Read the model definition and answer for the solid it produces. Units are mm, in the model's axes. A direction names the side the tool comes from. Round coordinates to 2 decimals unless told otherwise and drop trailing zeros. Order: outer loops, then holes, each group sorted by start corner. A loop starts at its lowest first (then second) coordinate and runs counter-clockwise, first axis right, second up. Notation, with made-up numbers: (3, 25.5) - (37, 25.5) arc R20 cw to (37, 41.5) - close; hole circle Ø4 at (-7, 49). An arc over 180 degrees is marked (long way). Put each result on its own line as item: value. Start each with the question number.
Q1. For a pull along Z with two mould halves and no side action, classify faces 1 (the face through (1.2, 6.4, -10.4)), 2 (the face through (15.62, 6.41, 3.47)), 3 (the face through (10, 0, -3)), 4 (the face through (1.2, 6.4, 13.6)) as pulls with the +Z half, pulls with the -Z half, needs draft (parallel to the pull), parting line crosses it, or undercut.
Q2. Section A-A on x = -12 is taken. Give the vertices of the cut face in (y, z).
Q3. Section B-B on y = 9.75 is taken. Give the vertices of the cut face in (x, z).
Q4. Which of the six approach directions +Z, -Z, +X, -X, +Y, -Y give full straight-line access (tool end or side, diameter ignored) to faces 5 (the face through (-9.76, -5.07, -2.17)), 6 (the face through (-4, 13, 4))?
Q5. Find the intervals of material crossed by line 1 along X through (y, z) = (7.5, 0); line 2 along X through (y, z) = (6, -0.5); line 3 along X through (y, z) = (-0.75, -1), in increasing order. Write a range as from..to.
Q6. Section C-C on z = 3 is taken. Give the vertices of the cut face in (x, y).
Q7. Each of these flat-tipped pins is pushed along its axis until it touches: pin 1 Ø13 at (x, z) = (0, 0) entering from -Y; pin 2 Ø2 at (y, z) = (-5, 1.5) entering from -X; pin 3 Ø2.5 at (x, z) = (0, -12) entering from +Y; pin 4 Ø5 at (y, z) = (3, 4) entering from +X. Where does it stop, or does it pass through?
Q8. Section D-D on z = -6.5 is taken. Give the vertices of the cut face in (x, y), then the cut area to 3 significant figures.
from build123d import *

# Parameters (mm, degrees)
SKETCH_1_R      = 16
SKETCH_1_R_2    = 2
SKETCH_1_R_3    = 5
EXTRUDE_1_DEPTH = 13
EXTRUDE_START   = -10
SKETCH_1_3_R    = 10
SKETCH_1_3_R_2  = 5
EXTRUDE_2_DEPTH = 10


with BuildPart() as part:
    # Sketch 1 → Extrude 1 (new body)
    with BuildSketch(Plane(origin=(0, 0, 0), x_dir=(1, 0, 0), z_dir=(0, 1, 0))):
        with Locations(Location((0, 0, 0), (0, 0, 90))):
            Circle(SKETCH_1_R)
        with Locations(Location((0, 12, 0), (0, 0, 90))):
            Circle(SKETCH_1_R_2, mode=Mode.SUBTRACT)
        with Locations(Location((12, 0, 0), (0, 0, 90))):
            Circle(SKETCH_1_R_2, mode=Mode.SUBTRACT)
        with Locations(Location((0, -12, 0), (0, 0, 90))):
            Circle(SKETCH_1_R_2, mode=Mode.SUBTRACT)
        with Locations(Location((-12, 0, 0), (0, 0, 90))):
            Circle(SKETCH_1_R_2, mode=Mode.SUBTRACT)
        with Locations(Location((0, 0, 0), (0, 0, 90))):
            Circle(SKETCH_1_R_3, mode=Mode.SUBTRACT)
    extrude(amount=EXTRUDE_1_DEPTH)

    # Sketch 1_3 → Extrude 2 (add)
    with BuildSketch(Plane(origin=(0, 0, 0), x_dir=(1, 0, 0), z_dir=(0, 1, 0)).offset(EXTRUDE_START)):
        with Locations(Location((0, 0, 0), (0, 0, 270))):
            Circle(SKETCH_1_3_R)
        with Locations(Location((0, 0, 0), (0, 0, 90))):
            Circle(SKETCH_1_3_R_2, mode=Mode.SUBTRACT)
    extrude(amount=EXTRUDE_2_DEPTH)


solid = part.part
Findings:
1. face 1: undercut
1. face 2: parting line crosses it
1. face 3: needs draft
1. face 4: undercut
2. outline: (0, -10.58) - (13, -10.58) - (13, -2) - (0, -2) - close; (0, 2) - (13, 2) - (13, 10.58) - (0, 10.58) - close
3. outline: circle Ø32 at (0, 0); hole circle Ø4 at (-12, 0); hole circle Ø10 at (0, 0); hole circle Ø4 at (0, -12); hole circle Ø4 at (0, 12); hole circle Ø4 at (12, 0)
4. face 5: -Y
4. face 6: +Z, -Z, +X, -X, +Y
5. line 1: -16..-14, -10..-5, 5..10, 14..16
5. line 2: -15.99..-13.94, -10.06..-4.97, 4.97..10.06, 13.94..15.99
5. line 3: -9.95..-4.9, 4.9..9.95
6. outline: (-15.72, 0) - (-9.54, 0) - (-9.54, -10) - (-4, -10) - (-4, 13) - (-15.72, 13) - close; (4, -10) - (9.54, -10) - (9.54, 0) - (15.72, 0) - (15.72, 13) - (4, 13) - close
7. pin 1: y = -10
7. pin 2: x = -9.99
7. pin 3: through
7. pin 4: x = 15.93
8. outline: (-14.62, 0) - (-7.6, 0) - (-7.6, -10) - (7.6, -10) - (7.6, 0) - (14.62, 0) - (14.62, 13) - (-14.62, 13) - close
8. area: 532 mm2
